```python
from build123d import *

# Parameters (mm, degrees)
ESQUISSE1_R             = 1.5
ESQUISSE1_W             = 4
ESQUISSE1_H             = 4
BOSS_EXTRU_1_DEPTH      = 4
ENL_V_MAT_EXTRU_1_REACH = 28.467


with BuildPart() as part:
    # Esquisse1 → Boss.-Extru.1 (new body)
    with BuildSketch(Plane.XY):
        with BuildLine():
            Line((-3.5, 0), (-3.5, 10))
            ThreePointArc((-3.5, 10), (-3.939339828, 11.060660172), (-5, 11.5))
            Line((-5, 11.5), (-15, 11.5))
            ThreePointArc((-15, 11.5), (-18.5, 15), (-15, 18.5))
            Line((-15, 18.5), (15, 18.5))
            ThreePointArc((15, 18.5), (18.5, 15), (15, 11.5))
            Line((15, 11.5), (5, 11.5))
            ThreePointArc((5, 11.5), (3.939339828, 11.060660172), (3.5, 10))
            Line((3.5, 10), (3.5, 0))
            ThreePointArc((3.5, 0), (0, -3.5), (-3.5, 0))
        make_face()
        Circle(ESQUISSE1_R, mode=Mode.SUBTRACT)
        with Locations((-15, 15)):
            Circle(ESQUISSE1_R, mode=Mode.SUBTRACT)
        with Locations((15, 15)):
            Circle(ESQUISSE1_R, mode=Mode.SUBTRACT)
        with Locations((-7, 15)):
            Rectangle(ESQUISSE1_W, ESQUISSE1_H, mode=Mode.SUBTRACT)
        with Locations((7, 15)):
            Rectangle(ESQUISSE1_W, ESQUISSE1_H, mode=Mode.SUBTRACT)
    extrude(amount=BOSS_EXTRU_1_DEPTH)

    # Esquisse2 → Enlèv. mat.-Extru.1 (cut, up to next)
    with BuildSketch(Plane.XY.offset(4), mode=Mode.PRIVATE) as enl_v_mat_extru_1_sk1:
        with BuildLine():
            Line((-1, 4.5), (-1, 15.5))
            ThreePointArc((-1, 15.5), (0, 16.5), (1, 15.5))
            Line((1, 15.5), (1, 4.5))
            ThreePointArc((1, 4.5), (0, 3.5), (-1, 4.5))
        make_face()
    enl_v_mat_extru_1_tool1 = extrude(enl_v_mat_extru_1_sk1.sketch, amount=-ENL_V_MAT_EXTRU_1_REACH, mode=Mode.PRIVATE) & part.part
    add(enl_v_mat_extru_1_tool1.solids().sort_by_distance((0, 10, 4))[0], mode=Mode.SUBTRACT)


solid = part.part
```
Input: part model. Units: mm. Frame: model coordinates. A direction names the side the tool comes from. Round coordinates to 2 decimals unless told otherwise and drop trailing zeros. Order: outer loops, then holes, each group sorted by start corner. A loop starts at its lowest first (then second) coordinate and runs counter-clockwise, first axis right, second up. Notation, with made-up numbers: (78.25, 4.5) - (118.25, 4.5) arc R17 cw to (118.25, 13.5) - close; hole circle Ø6 at (14.5, 15.5). An arc over 180 degrees is marked (long way). Answer in a Markdown table with one row per item.
Item 1: Mould query, pull axis X, two halves, no side actions, for faces 1 (the flat face through (5, 15, 2)), 2 (the cylindrical face through (0.1, -3.5, 2)), 3 (the flat face through (-1.3, 12.4, 0)). Classes: released by +X, released by -X, zero draft, split by the parting line, or undercut.
Model answer:
| item | result |
|---|---|
| face 1 | undercut |
| face 2 | split by the parting line |
| face 3 | zero draft |
Item 2: Section query D-D (z = 1.8). Return the cut outline in (x, y), then the cut area to 3 significant figures.
Model answer:
| item | result |
|---|---|
| outline | (-15, 11.5) - (-5, 11.5) arc R1.5 cw to (-3.5, 10) - (-3.5, 0) arc R3.5 ccw to (3.5, 0) - (3.5, 10) arc R1.5 cw to (5, 11.5) - (15, 11.5) arc R3.5 ccw to (15, 18.5) - (-15, 18.5) arc R3.5 ccw to start; hole circle Ø3 at (-15, 15); hole (-9, 13) - (-5, 13) - (-5, 17) - (-9, 17) - close; hole circle Ø3 at (0, 0); hole (-1, 4.5) arc R1 ccw to (1, 4.5) - (1, 15.5) arc R1 ccw to (-1, 15.5) - close; hole (5, 13) - (9, 13) - (9, 17) - (5, 17) - close; hole circle Ø3 at (15, 15) |
| area | 271 mm² |
Item 3: Reachability of faces 4 (the flat face through (1, 10, 2)), 5 (the flat face through (0, 18.5, 2)), 6 (the flat face through (3.5, 5, 2)) from +Z, -Z, +X, -X, +Y, -Y: full face, straight path, thin tool, end or side. Return the list, or none.
Model answer:
| item | result |
|---|---|
| face 4 | +Z, -Z |
| face 5 | +Z, -Z, +X, -X, +Y |
| face 6 | +Z, -Z, +X, -Y |
Item 4: Section query C-C (x = 0). Return the cut outline in (y, z), then the cut area to 3 significant figures.
Model answer:
| item | result |
|---|---|
| outline | (-3.5, 0) - (-1.5, 0) - (-1.5, 4) - (-3.5, 4) - close; (1.5, 0) - (3.5, 0) - (3.5, 4) - (1.5, 4) - close; (16.5, 0) - (18.5, 0) - (18.5, 4) - (16.5, 4) - close |
| area | 24.0 mm² |
Item 5: Section query B-B (y = 7). Return the cut outline in (x, z), then the cut area to 3 significant figures.
Model answer:
| item | result |
|---|---|
| outline | (-3.5, 0) - (-1, 0) - (-1, 4) - (-3.5, 4) - close; (1, 0) - (3.5, 0) - (3.5, 4) - (1, 4) - close |
| area | 20.0 mm² |
Item 6: Line query: line 1 (Y direction, x = 0, z = 1.35); line 2 (Y direction, x = 15, z = 3.7); line 3 (X direction, y = 5.75, z = 2.55). Output: solid intervals per line, ascending.
Model answer:
| item | result |
|---|---|
| line 1 | y = -3.5 to -1.5, 1.5 to 3.5, 16.5 to 18.5 |
| line 2 | y = 11.5 to 13.5, 16.5 to 18.5 |
| line 3 | x = -3.5 to -1, 1 to 3.5 |
Item 7: Section query A-A (x = 7.5). Return the cut outline in (y, z).
Model answer:
| item | result |
|---|---|
| outline | (11.5, 0) - (13, 0) - (13, 4) - (11.5, 4) - close; (17, 0) - (18.5, 0) - (18.5, 4) - (17, 4) - close |
Item 8: Pin query (flat end, axial travel): pin 1 (2.5 mm diameter, centred on x = -15, y = 15, fed in from -Z); pin 2 (2 mm diameter, centred on y = 7.5, z = 1.5, fed in from +X); pin 3 (1 mm diameter, centred on y = 11.5, z = 2.5, fed in from +X); pin 4 (1.2 mm diameter, centred on x = 8.5, z = 1.5, fed in from -Y). Return the tip coordinate at first contact, or that it passes through.
Model answer:
| item | result |
|---|---|
| pin 1 | passes through |
| pin 2 | stops at x = 3.5 |
| pin 3 | stops at x = 16.8 |
| pin 4 | stops at y = 11.5 |
